from build123d import *

# Parameters (mm, degrees)
SKETCH1_W           = 20
SKETCH1_H           = 31
SKETCH1_W_2         = 12
SKETCH1_H_2         = 21
BOSS_EXTRUDE1_DEPTH = 6.5
CHAMFER1_SIZE       = 2


with BuildPart() as part:
    # Sketch1 → Boss-Extrude1 (new body)
    with BuildSketch(Plane.XY):
        Rectangle(SKETCH1_W, SKETCH1_H)
        Rectangle(SKETCH1_W_2, SKETCH1_H_2, mode=Mode.SUBTRACT)
    extrude(amount=BOSS_EXTRUDE1_DEPTH)

    # Chamfer1
    chamfer1_edges = [part.edges().sort_by_distance(p)[0] for p in [
        (10, -15.5, 3.25),
        (-10, -15.5, 3.25),
        (-10, 15.5, 3.25),
        (10, 15.5, 3.25),
    ]]
    chamfer(chamfer1_edges, length=CHAMFER1_SIZE)


solid = part.part
The model under review builds one solid part; all positions refer to its coordinate system, in mm. A direction names the side the tool comes from. Give positions to 0.01 mm unless a question says otherwise; leave off trailing zeros. Loops run counter-clockwise (first coordinate to the right, second up) from the corner with the lowest first, then second, coordinate; pieces in that order, holes last. Notation, with made-up numbers: (43.5, 47.5) -> (98.5, 47.5) arc R36 ccw to (98.5, 85.5) -> close; hole circle Ø2 at (87, 76.25). An arc over 180 degrees is marked (long way). Answer as a JSON object with one key per item and string values. Group by question number.
Q1. Wall thickness on line 1 along X through (y, z) = (8.5, 2.75); line 2 along Y through (x, z) = (-2.5, 5.5); line 3 along Y through (x, z) = (8.25, 0.5): over which ranges is each line inside the solid? List them lowest first.
Q2. Take a section at A-A (y = -7). Write out the cut boundary in (x, z), plus the area to 3 significant figures.
Q3. Take a section at C-C (z = 5.75). Write out the cut boundary in (x, y), plus the area to 3 significant figures.
Q4. Draft analysis for pull direction X (two halves, no side actions). For faces 1 (the flat face through (-6, 0, 3)), 2 (the flat face through (-9, -14.5, 3.2)), 3 (the flat face through (0, 15.5, 3)), 4 (the flat face through (9, -14.5, 3.2)), state which applies: pulls with the +X half, pulls with the -X half, needs draft (parallel to the pull), parting line crosses it, or undercut.
Q5. Take a section at B-B (x = 4). Write out the cut boundary in (y, z).
Q6. Tool access review of faces 5 (the flat face through (0, -10.5, 3)), 6 (the flat face through (10, 0, 3)): name each direction out of +Z, -Z, +X, -X, +Y, -Y from which nothing blocks a thin tool from reaching the whole face with its end or side.
Answer below:
{
 "1": {"line 1": "x = -10 to -6, 6 to 10", "line 2": "y = -15.5 to -10.5, 10.5 to 15.5", "line 3": "y = -15.25 to 15.25"},
 "2": {"outline": "(-10, 0) -> (-6, 0) -> (-6, 6.5) -> (-10, 6.5) -> close; (6, 0) -> (10, 0) -> (10, 6.5) -> (6, 6.5) -> close", "area": "52.0 mm2"},
 "3": {"outline": "(-10, -13.5) -> (-8, -15.5) -> (8, -15.5) -> (10, -13.5) -> (10, 13.5) -> (8, 15.5) -> (-8, 15.5) -> (-10, 13.5) -> close; hole (-6, -10.5) -> (6, -10.5) -> (6, 10.5) -> (-6, 10.5) -> close", "area": "360 mm2"},
 "4": {"face 1": "undercut", "face 2": "pulls with the -X half", "face 3": "needs draft", "face 4": "pulls with the +X half"},
 "5": {"outline": "(-15.5, 0) -> (-10.5, 0) -> (-10.5, 6.5) -> (-15.5, 6.5) -> close; (10.5, 0) -> (15.5, 0) -> (15.5, 6.5) -> (10.5, 6.5) -> close"},
 "6": {"face 5": "+Z, -Z", "face 6": "+Z, -Z, +X, +Y, -Y"}
}
